Autodesk Inventor part; units mm, degrees
ref_plane "YZ Plane" through (0, 0, 0) normal (1, 0, 0) x (0, 1, 0)
ref_plane "XZ Plane" through (0, 0, 0) normal (0, 1, 0) x (-1, 0, 0)
ref_plane "XY Plane" through (0, 0, 0) normal (0, 0, 1) x (1, 0, 0)
sketch "Эскиз5" plane through (0, 0, 0) normal (0, 0, 1) x (1, 0, 0)
  line L0 (0, 0) -> (20, 0)
  line L1 (20, 0) -> (20, 25)
  line L2 (16, 29) -> (4, 29)
  line L3 (0, 25) -> (0, 0)
  line L4 (4, 29) -> (0, 25)
  line L5 (16, 29) -> (20, 25)
  point P0 (20, 29)
  point P1 (0, 29)
  dimension "d33" = 20
  dimension "d34" = 29
  dimension "d35" = 4
  dimension "d36" = 4
  dimension "d37" = 4
  dimension "d38" = 4
revolve "Вращение3" add sketch "Эскиз5" angle 360 about axis through (0, 0, 0) along (1, 0, 0)
sketch "Эскиз6" plane through (0, 0, 0) normal (0, 0, 1) x (1, 0, 0)
  line L0 (0, -25) -> (0, 25) construction
  line L1 (0, 4) -> (9, 4)
  line L2 (9, 4) -> (9, -4)
  line L3 (9, -4) -> (0, -4)
  line L4 (0, -4) -> (0, 4)
  point P0 (0, 0)
  point P1 (0, 0)
  point P2 (0, 0)
  dimension "d40" = 9
  dimension "d41" = 8
extrude "Выдавливание2" cut sketch "Эскиз6" along normal through all both and the other way through all
sketch "Эскиз7" plane through (0, 0, 0) normal (-1, 0, 0) x (0, 0, 1)
  line L0 (0, 0) -> (0, 23) construction
  dimension "d44" = 23
hole "Отверстие2" at (0, 23, 0) direction (1, 0, 0) diameter 4 end through all
sketch "Эскиз8" plane through (20, 0, 0) normal (1, 0, 0) x (0, 0, -1)
  point P0 (0, 0)
  point P1 (0, 0)
hole "Отверстие3" at (20, 0, 0) direction (-1, 0, 0) diameter 8 depth 5
sketch "Эскиз9" plane through (15, 0, 0) normal (1, 0, 0) x (0, 0, -1)
  circle A0 centre (0, 0) radius 4.5
  dimension "d59" = 9
extrude "Выдавливание3" cut sketch "Эскиз9" against normal blind 0.5
thread "Резьба2"
properties part number "711134"
For this review, take the finished solid that the model builds, in its own axes (mm). A direction names the side the tool comes from. Coordinates: 2 decimals unless noted, no trailing zeros. Order: outer loops, then holes, each group sorted by start corner. A loop starts at its lowest first (then second) coordinate and runs counter-clockwise, first axis right, second up. Notation, with made-up numbers: (-16.5, 56) -> (-3.5, 56) arc R13 cw to (-3.5, 66) -> close; hole circle Ø8 at (51, 79). An arc over 180 degrees is marked (long way). Use CSV: the item, a comma, the result in double quotes. Start each with the question number.
Item 1: We need section A-A, the plane x = 6.25. Give the boundary of the cut face in (y, z), then the cut area to 3 significant figures.
Item 2: Wall thickness on probe 1 along Y at (x, z) = (14.7, 0); probe 2 along Y at (x, z) = (4.75, 0); probe 3 along Y at (x, z) = (10.25, 0): over which ranges is each line inside the solid? List them lowest first.
Item 3: Draft analysis for pull direction Y (two halves, no side actions). For faces 4 (the face through (20, 0, -5)), 5 (the face through (17.465, 3.905, 0.867)), 6 (the face through (0.25, -25.245, 0.506)), 7 (the face through (14.5, 0, 0)), state which applies: pulls with the +Y half, pulls with the -Y half, needs draft (parallel to the pull), parting line crosses it, or undercut.
Item 4: For faces 1 (the face through (5, -4, 0)), 2 (the face through (15, -3, 3)), 3 (the face through (0, 12, 0)), list the 3-axis set-ups (+Z, -Z, +X, -X, +Y, -Y) from which the entire face can be reached by the end or side of a thin tool; tool diameter is ignored.
Item 5: We need section C-C, the plane x = 3. Give the boundary of the cut face in (y, z), then the cut area to 3 significant figures.
Item 6: We need section B-B, the plane y = 0. Give the boundary of the cut face in (x, z).
Item 7: Insertion check: pin 1 (5 mm diameter, centred on x = 9.5, z = -21, fed in from +Y); pin 2 (7 mm diameter, centred on y = 0, z = 0, fed in from -X); pin 3 (6 mm diameter, centred on x = 3.5, z = -19.5, fed in from -Y). Each pin has a flat end and moves straight along its axis. Give the tip position at first contact, or say it passes through.
Derived:
1,outline,"(-4, -28.72) -> (-4, 28.72) arc R29 ccw to start; (4, -28.72) arc R29 ccw to (4, 28.72) -> close; hole circle Ø4 at (23, 0)"
1,area,"2,170 mm^2"
2,probe 1,"y = -29 to -4.5, 4.5 to 21, 25 to 29"
2,probe 2,"y = -29 to -4, 4 to 21, 25 to 29"
2,probe 3,"y = -29 to 21, 25 to 29"
3,face 4,"needs draft"
3,face 5,"undercut"
3,face 6,"pulls with the -Y half"
3,face 7,"undercut"
4,face 1,"+Z, -Z, -X"
4,face 2,"none"
4,face 3,"+Z, -Z, -X, +Y, -Y"
5,outline,"(-4, -27.71) -> (-4, 27.71) arc R28 ccw to start; (4, -27.71) arc R28 ccw to (4, 27.71) -> close; hole circle Ø4 at (23, 0)"
5,area,"2,000 mm^2"
6,outline,"(9, -29) -> (16, -29) -> (20, -25) -> (20, -4) -> (15, -4) -> (15, -4.5) -> (14.5, -4.5) -> (14.5, 4.5) -> (15, 4.5) -> (15, 4) -> (20, 4) -> (20, 25) -> (16, 29) -> (9, 29) -> close"
7,pin 1,"stops at y = 22.33"
7,pin 2,"stops at x = 9"
7,pin 3,"stops at y = -23.82"
